```python
from build123d import *

# Parameters (mm, degrees)
F1_DEPTH = 10
F2_R     = 10.5
F3_DEPTH = 5.5
F4_R     = 10
F5_DEPTH = 16
F6_SIZE  = 1
F8_D     = 8.8


with BuildPart() as f1:
    # F0 (on Top) → F1 (new body)
    with BuildSketch(Plane.XY):
        Polygon((3.5951366344, -13.3818904711), (13.3866254158, -3.5774655801), (9.7914887815, 9.804424891), (-3.5951366344, 13.3818904711), (-13.3866254158, 3.5774655801), (-9.7914887815, -9.804424891), align=None)
    extrude(amount=F1_DEPTH)

    # F2 (on face) → F3 (join)
    with BuildSketch(Plane.XY.offset(10)):
        Circle(F2_R)
    extrude(amount=F3_DEPTH)

    # F4 (on face) → F5 (join)
    with BuildSketch(Plane.XY.offset(15.5)):
        Circle(F4_R)
    extrude(amount=F5_DEPTH)

    # F6
    f6_edges = [f1.edges().sort_by_distance(p)[0] for p in [
        (-10, 0, 31.5),
    ]]
    chamfer(f6_edges, length=F6_SIZE)

    # F8 (through all)
    with Locations(Plane(origin=(0, 0, 0), x_dir=(1, 0, 0), z_dir=(0, 0, -1))):
        with Locations((0, 0)):
            Hole(F8_D / 2)


solid = f1.part
```
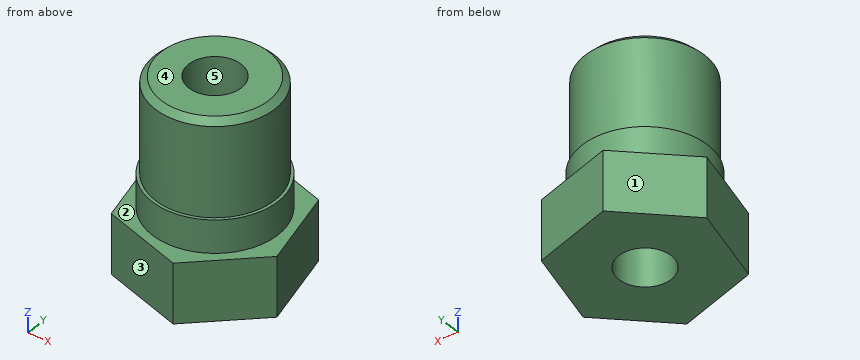
For this review, take the finished solid that the model builds, in its own axes (mm). Face numbers are marked on the shaded views. A direction names the side the tool comes from. Round coordinates to 2 decimals unless told otherwise and drop trailing zeros. Write each loop counter-clockwise with the first axis right and the second up, starting at its lowest first coordinate (ties: lowest second). Pieces come first, ordered by that corner, then holes. Notation, with made-up numbers: (78, 80) - (125, 80) arc R17 cw to (125, 84) - close; hole circle Ø6 at (14, 49.25). An arc over 180 degrees is marked (long way). Put each result on its own line as item: value.
Q1. Machinability: for the marked faces 1 and 2, which of the approach directions +Z, -Z, +X, -X, +Y, -Y give a long, thin tool a straight path to every point of the face, cutting with its end or side? Answer none if there is none.
Solved:
face 1: +Z, -Z, -X, +Y
face 2: +Z
Q2. Mouldability with a two-part tool opening along Y and no side actions: class the marked faces 3, 4 and 5 as released by +Y, released by -Y, zero draft, split by the parting line, or undercut.
Solved:
face 3: released by -Y
face 4: zero draft
face 5: undercut
Q3. We need section D-D (z = 14). Give the boundary of the cut face in (x, y).
Solved:
outline: circle Ø21 at (0, 0); hole circle Ø8.8 at (0, 0)
Q4. We need section C-C (x = 0). Give the boundary of the cut face in (y, z), and give its area (3 significant figures).
Solved:
outline: (-12.42, 0) - (-4.4, 0) - (-4.4, 31.5) - (-9, 31.5) - (-10, 30.5) - (-10, 15.5) - (-10.5, 15.5) - (-10.5, 10) - (-12.42, 10) - close; (4.4, 0) - (12.42, 0) - (12.42, 10) - (10.5, 10) - (10.5, 15.5) - (10, 15.5) - (10, 30.5) - (9, 31.5) - (4.4, 31.5) - close
area: 406 mm2
Q5. Wall thickness on probe 1 along Y at (x, z) = (0, 12); probe 2 along Y at (x, z) = (0, 17); probe 3 along Z at (x, y) = (-4.25, 9.75): over which ranges is each line inside the solid? List them lowest first.
Solved:
probe 1: y = -10.5 to -4.4, 4.4 to 10.5
probe 2: y = -10 to -4.4, 4.4 to 10
probe 3: z = 0 to 10
Q6. Insertion check: pin 1 Ø1.5 at (y, z) = (-8.5, 11) entering from -X; pin 2 Ø6 at (y, z) = (8, 4.5) entering from +X; pin 3 Ø6 at (x, z) = (-0.5, 12) entering from +Y. Each pin has a flat end and moves straight along its axis. Give the tip position at first contact, or say it passes through.
Solved:
pin 1: stops at x = -7.08
pin 2: stops at x = 11.08
pin 3: stops at y = 13.15
Q7. We need section B-B (y = 0). Give the boundary of the cut face in (x, z), and give its area (3 significant figures).
Solved:
outline: (-12.43, 0) - (-4.4, 0) - (-4.4, 31.5) - (-9, 31.5) - (-10, 30.5) - (-10, 15.5) - (-10.5, 15.5) - (-10.5, 10) - (-12.43, 10) - close; (4.4, 0) - (12.43, 0) - (12.43, 10) - (10.5, 10) - (10.5, 15.5) - (10, 15.5) - (10, 30.5) - (9, 31.5) - (4.4, 31.5) - close
area: 406 mm2
Q8. We need section A-A (z = 2.5). Give the boundary of the cut face in (x, y).
Solved:
outline: (-13.39, 3.58) - (-9.79, -9.8) - (3.6, -13.38) - (13.39, -3.58) - (9.79, 9.8) - (-3.6, 13.38) - close; hole circle Ø8.8 at (0, 0)
